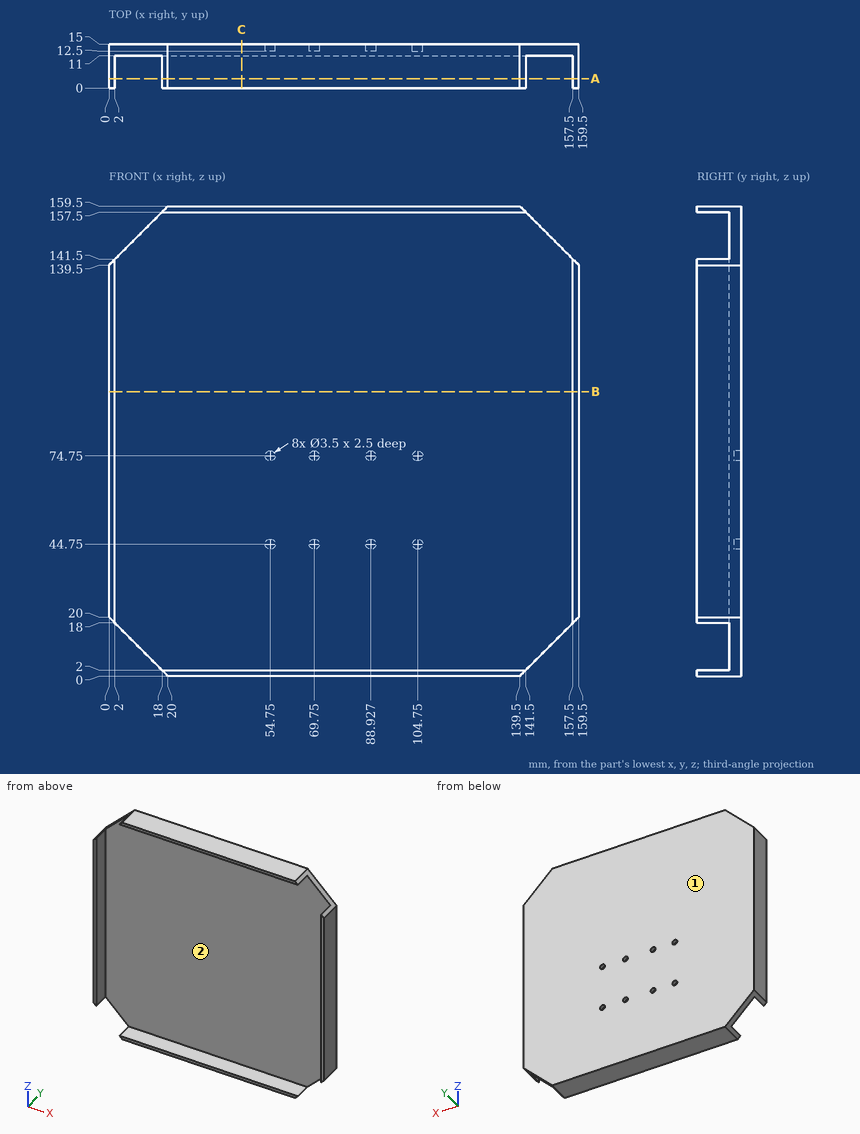
Could you check a few things on this drawing? It's one solid part, dimensions in mm from its lowest x, y, z. Coordinates: 2 decimals unless noted, no trailing zeros. Order: outer loops, then holes, each group sorted by start corner. A loop starts at its lowest first (then second) coordinate and runs counter-clockwise, first axis right, second up. Notation, with made-up numbers: M 17.5,89 L 48.5,89 A21 cw 48.5,125 Z; hole C 41.5,31 d7. An arc over 180 degrees is marked long. Use a Markdown table: item, result. Add a question column.
Q1. I want a section at C-C on x = 45. List the corners of the cut face in (y, z) for me, then the cut area to 3 significant figures.
Q2. We'd pull the mould along X, two halves only. Please class the marked faces 1 and 2: pulls with the +X half, pulls with the -X half, needs draft (parallel to the pull), parting line crosses it, or undercut.
Q3. I'm going to push flat-ended pins straight in: pin 1 (12 mm diameter, centred on x = 123.5, z = 43.5, fed in from -Y); pin 2 (1 mm diameter, centred on x = 104, z = 45, fed in from +Y). Where does each tip first touch, or does it pass through?
Q4. If I drill on L1, parallel to X at y = 14.1, z = 44.75; L2, parallel to Z at x = 104.75, y = 13; L3, parallel to X at y = 3.5, z = 20.5, over which ranges is the centre line in solid material (lowest first)?
Q5. I want a section at A-A on y = 3.25. List the corners of the cut face in (x, z) for me.
Q6. I want a section at B-B on z = 96.5. List the corners of the cut face in (x, y) for me, then the cut area to 3 significant figures.
Checked values:
| question | item | result |
|---|---|---|
| 1 | outline | M 0,0 L 15,0 L 15,159.5 L 0,159.5 L 0,157.5 L 11,157.5 L 11,2 L 0,2 Z |
| 1 | area | 682 mm² |
| 2 | face 1 | needs draft |
| 2 | face 2 | undercut |
| 3 | pin 1 | y = 11 |
| 3 | pin 2 | y = 12.5 |
| 4 | L1 | 0 to 53, 56.5 to 68, 71.5 to 87.18, 90.68 to 103, 106.5 to 159.5 |
| 4 | L2 | 0 to 43, 46.5 to 73, 76.5 to 159.5 |
| 4 | L3 | 0 to 2, 157.5 to 159.5 |
| 5 | outline | M 0,20 L 2,18 L 2,141.5 L 0,139.5 Z; M 18,2 L 20,0 L 139.5,0 L 141.5,2 Z; M 18,157.5 L 141.5,157.5 L 139.5,159.5 L 20,159.5 Z; M 157.5,18 L 159.5,20 L 159.5,139.5 L 157.5,141.5 Z |
| 6 | outline | M 0,0 L 2,0 L 2,11 L 157.5,11 L 157.5,0 L 159.5,0 L 159.5,15 L 0,15 Z |
| 6 | area | 682 mm² |
